The model under review builds one solid part; all positions refer to its coordinate system, in mm. A direction names the side the tool comes from. Round coordinates to 2 decimals unless told otherwise and drop trailing zeros. Answer as a JSON object with one key per item and string values. Group by question number.
1) To check wall thickness, follow line 1 (Y direction, x = -4.1, z = 0); line 2 (X direction, y = 31, z = -2.5) (3 decimals); line 3 (Y direction, x = -3.95, z = 0). State the ranges of each line that lie inside material, in increasing order.
2) For faces 1 (the flat face through (-3.375, 30.7, 2)), 2 (the flat face through (4.5, 35, -3)), 3 (the flat face through (3.375, 31, 4)), list the 3-axis set-ups (+Z, -Z, +X, -X, +Y, -Y) from which the entire face can be reached by the end or side of a thin tool; tool diameter is ignored.
3) Insertion check: pin 1 Ø1 at (x, z) = (-3, -4) entering from -Y; pin 2 Ø2 at (x, y) = (1, 15) entering from -Z; pin 3 Ø5 at (x, z) = (-2.5, 2) entering from +Y; pin 4 Ø5 at (y, z) = (36, 0) entering from +X. Each pin has a flat end and moves straight along its axis. Give the tip position at first contact, or say it passes through.
```python
from build123d import *

# Parameters (mm, degrees)
WYTNIJ_WYCI_GNI_CIE1_DEPTH      = 10.998876849
WYTNIJ_WYCI_GNI_CIE1_DEPTH_BACK = 10.998876849
SZKIC4_W                        = 1.45
SZKIC4_H                        = 9
SZKIC8_R                        = 3
WYTNIJ_WYCI_GNI_CIE3_DEPTH      = 5.5
WYTNIJ_WYCI_GNI_CIE3_DEPTH_BACK = 5.5


with BuildPart() as part:
    # Szkic1 one side → Obrót4 (revolve)
    with BuildSketch(Plane.XY):
        with BuildLine():
            Line((-3, 21), (-3, 0))
            Line((-3, 0), (0, 0))
            Line((0, 0), (0.005166955, 46))
            ThreePointArc((0.005166955, 46), (-8.632770826, 41.038455208), (-8.699205566, 31.077206177))
            Line((-8.699205566, 31.077206177), (-3, 21))
        make_face()
    revolve(axis=Axis((0.005166955, 46, 0), (-0.000112325, -0.999999994, 0)))

    # Szkic2 → Wytnij-wyciągnięcie1 (cut, two sides)
    with BuildSketch(Plane.XY) as wytnij_wyci_gni_cie1_sk:
        Polygon((-3.375, 46), (-20, 46), (-20, 10.866665268), (-3.375, 21.663066505), align=None)
        Polygon((20, 46), (3.375, 46), (3.375, 21.65370739), (20, 10.857306153), align=None)
    extrude(amount=WYTNIJ_WYCI_GNI_CIE1_DEPTH, mode=Mode.SUBTRACT)
    extrude(wytnij_wyci_gni_cie1_sk.sketch, amount=-WYTNIJ_WYCI_GNI_CIE1_DEPTH_BACK, mode=Mode.SUBTRACT)

    # Szkic4 → Obrót5 (revolve)
    with BuildSketch(Plane.YX):
        with BuildLine():
            Line((40.449326049, 4.5), (40.449326049, -4.5))
            ThreePointArc((40.449326049, -4.5), (41.839498769, -2.438212993), (42.328030498, 0))
            ThreePointArc((42.328030498, 0), (41.839498769, 2.438212993), (40.449326049, 4.5))
        make_face()
        with Locations((39.724326049, 0)):
            Rectangle(SZKIC4_W, SZKIC4_H)
    revolve(axis=Axis((-0.999999975, 35.999326049, 0), (1, 0, 0)))

    # Szkic8 → Wytnij-wyciągnięcie3 (cut, two sides)
    with BuildSketch(Plane(origin=(0, 0, 0), x_dir=(0, 0, -1), z_dir=(1, 0, 0))) as wytnij_wyci_gni_cie3_sk:
        with Locations((0, 35.999326049)):
            Circle(SZKIC8_R)
    extrude(amount=WYTNIJ_WYCI_GNI_CIE3_DEPTH, mode=Mode.SUBTRACT)
    extrude(wytnij_wyci_gni_cie3_sk.sketch, amount=-WYTNIJ_WYCI_GNI_CIE3_DEPTH_BACK, mode=Mode.SUBTRACT)


solid = part.part
```
Results list:
{
 "1": {"line 1": "31.18 to 33, 39 to 40.82", "line 2": "-3.375 to 3.375", "line 3": "31.05 to 33, 39 to 40.94"},
 "2": {"face 1": "-X", "face 2": "+Z, -Z, +X, +Y, -Y", "face 3": "+X"},
 "3": {"pin 1": "y = 23.65", "pin 2": "z = -3", "pin 3": "y = 45.98", "pin 4": "through"}
}
